Build history of the part. All positions in model axes, mm. A direction names the side the tool comes from. Round coordinates to 2 decimals unless told otherwise and drop trailing zeros. Write each loop counter-clockwise with the first axis right and the second up, starting at its lowest first coordinate (ties: lowest second). Pieces come first, ordered by that corner, then holes.
Item 1: Band-saw the part on D-D, the plane y = -9. Write the cut outline in (x, z).
Item 2: Band-saw the part on C-C, the plane y = -2. Write the cut outline in (x, z), then the cut area to 3 significant figures.
Item 3: Band-saw the part on B-B, the plane z = -55. Write the cut outline in (x, y), then the cut area to 3 significant figures.
Item 4: Band-saw the part on A-A, the plane x = 30. Write the cut outline in (y, z).
Item 5: Mould opens along Z. For faces 1 (the flat face through (17.4, 0.4, 0)), 2 (the cylindrical face through (0.986, -8.512, -86.282)), 3 (the flat face through (22, 1, -17)), 4 (the cylindrical face through (44.1, 1.14, -11.15)) say: +Z half, -Z half, draft (parallel to the pull), parting line (faces both ways), or undercut.
Item 6: Wall check: probe 1 along X at (y, z) = (-11.25, -5); probe 2 along Z at (x, y) = (0.9, -9); probe 3 along Z at (x, y) = (0.95, -9.5). Give the ranges that are in metal, low to high.
Item 7: Drop flat-ended pins along their axis: pin 1 Ø2 at (x, z) = (1, -49.5) entering from +Y; pin 2 Ø0.6 at (x, y) = (22, 1.5) entering from -Z; pin 3 Ø0.6 at (y, z) = (0.5, -14) entering from -X; pin 4 Ø12 at (x, z) = (11, -80) entering from +Y. Give the stop position or say it passes through.
Item 8: 3-axis set-ups, long thin cutter, end or side, ignore diameter. For faces 5 (the cylindrical face through (43.99, -9.12, -56.71)), 6 (the flat face through (2, -7.7, -54.2)), 7 (the cylindrical face through (44.014, -9.867, -93.905)): which of +Z, -Z, +X, -X, +Y, -Y reach the whole face in a straight line?
```python
from build123d import *

# Parameters (mm, degrees)
SKETCH1_W                      = 45
SKETCH1_H                      = 22
BASE_FLANGE1_DEPTH             = 2
EDGE_FLANGE3_STRIP_W           = 10
EDGE_FLANGE3_STRIP_H           = 2
EDGE_FLANGE3_STRIP_CUT_DEPTH   = 22
EDGE_FLANGE3_STRIP_2_W         = 10
EDGE_FLANGE3_STRIP_2_H         = 2
EDGE_FLANGE3_STRIP_CUT_2_DEPTH = 22
EDGE_FLANGE3_DEPTH             = 22
EDGE_FLANGE3_PROFILE_W         = 110
EDGE_FLANGE3_PROFILE_H         = 17
EDGE_FLANGE3_FLAT_DEPTH        = 2
EDGE_FLANGE3_BEND_DEPTH        = 22
EDGE_FLANGE3_PROFILE_2_W       = 110
EDGE_FLANGE3_PROFILE_2_H       = 17
EDGE_FLANGE3_FLAT_2_DEPTH      = 2
SKETCH34_R                     = 4
CUT_EXTRUDE1_DEPTH             = 10
SKETCH35_R                     = 3.75
CUT_EXTRUDE2_DEPTH             = 10
SKETCH36_R                     = 1.75
CUT_EXTRUDE3_DEPTH             = 121.203993278
SKETCH37_W                     = 23
SKETCH37_H                     = 12
CUT_EXTRUDE4_DEPTH             = 10
CHAMFER1_SIZE                  = 2
CHAMFER2_SIZE                  = 10


# Sheet-metal steps are written as plain solids
with BuildPart() as part:
    # Sketch1 → Base-Flange1 (new body)
    with BuildSketch(Plane(origin=(0, 0, 0), x_dir=(1, 0, 0), z_dir=(0, 1, 0))):
        with Locations((22.5, 11)):
            Rectangle(SKETCH1_W, SKETCH1_H)
    extrude(amount=BASE_FLANGE1_DEPTH)

    # Edge-Flange3 strip (across the edge) → Edge-Flange3 strip cut (cut)
    with BuildSketch(Plane(origin=(45, 0, -22), x_dir=(-1, 0, 0), z_dir=(0, 0, 1))):
        with Locations((-2, -1)):
            Rectangle(EDGE_FLANGE3_STRIP_W, EDGE_FLANGE3_STRIP_H)
    extrude(amount=EDGE_FLANGE3_STRIP_CUT_DEPTH, mode=Mode.SUBTRACT)

    # Edge-Flange3 strip 2 (across the edge) → Edge-Flange3 strip cut 2 (cut)
    with BuildSketch(Plane(origin=(0, 0, 0), x_dir=(1, 0, 0), z_dir=(0, 0, -1))):
        with Locations((-2, -1)):
            Rectangle(EDGE_FLANGE3_STRIP_2_W, EDGE_FLANGE3_STRIP_2_H)
    extrude(amount=EDGE_FLANGE3_STRIP_CUT_2_DEPTH, mode=Mode.SUBTRACT)

    # Edge-Flange3 bend section (across the edge) → Edge-Flange3 (add)
    with BuildSketch(Plane(origin=(45, 0, -22), x_dir=(-1, 0, 0), z_dir=(0, 0, 1))):
        with BuildLine():
            Line((0, 1), (2, 1))
            ThreePointArc((2, 1), (2.292893219, 0.292893219), (3, 0))
            Line((3, 0), (3, -2))
            ThreePointArc((3, -2), (0.878679656, -1.121320344), (0, 1))
        make_face()
    extrude(amount=EDGE_FLANGE3_DEPTH)

    # Edge-Flange3 profile (on flange) → Edge-Flange3 flat (add)
    with BuildSketch(Plane(origin=(45, 0, 0), x_dir=(0, 0, 1), z_dir=(1, 0, 0))):
        with Locations((-55, 9.5)):
            Rectangle(EDGE_FLANGE3_PROFILE_W, EDGE_FLANGE3_PROFILE_H)
    extrude(amount=-EDGE_FLANGE3_FLAT_DEPTH)

    # Edge-Flange3 bend section 2 (across the edge) → Edge-Flange3 bend (add)
    with BuildSketch(Plane(origin=(0, 0, 0), x_dir=(1, 0, 0), z_dir=(0, 0, -1))):
        with BuildLine():
            Line((0, 1), (2, 1))
            ThreePointArc((2, 1), (2.292893219, 0.292893219), (3, 0))
            Line((3, 0), (3, -2))
            ThreePointArc((3, -2), (0.878679656, -1.121320344), (0, 1))
        make_face()
    extrude(amount=EDGE_FLANGE3_BEND_DEPTH)

    # Edge-Flange3 profile 2 (on flange) → Edge-Flange3 flat 2 (add)
    with BuildSketch(Plane(origin=(0, 0, 0), x_dir=(0, 0, -1), z_dir=(-1, 0, 0))):
        with Locations((55, 9.5)):
            Rectangle(EDGE_FLANGE3_PROFILE_2_W, EDGE_FLANGE3_PROFILE_2_H)
    extrude(amount=-EDGE_FLANGE3_FLAT_2_DEPTH)

    # Sketch34 → Cut-Extrude1 (cut)
    with BuildSketch(Plane(origin=(45, 0, 0), x_dir=(0, 0, -1), z_dir=(1, 0, 0))):
        with Locations(Location((90, -9, 0), (0, 0, 90))):
            Circle(SKETCH34_R)
    extrude(amount=-CUT_EXTRUDE1_DEPTH, mode=Mode.SUBTRACT)

    # Sketch35 → Cut-Extrude2 (cut)
    with BuildSketch(Plane.ZY):
        with Locations(Location((-90, -9, 0), (0, 0, 270))):
            Circle(SKETCH35_R)
    extrude(amount=-CUT_EXTRUDE2_DEPTH, mode=Mode.SUBTRACT)

    # Sketch36 → Cut-Extrude3 (cut, through all)
    with BuildSketch(Plane.ZY):
        with Locations(Location((-55, -9.5, 0), (0, 0, 270))):
            Circle(SKETCH36_R)
    extrude(amount=-CUT_EXTRUDE3_DEPTH, mode=Mode.SUBTRACT)

    # Sketch37 → Cut-Extrude4 (cut)
    with BuildSketch(Plane(origin=(0, 2, 0), x_dir=(1, 0, 0), z_dir=(0, 1, 0))):
        with Locations((22.5, 11)):
            Rectangle(SKETCH37_W, SKETCH37_H)
    extrude(amount=-CUT_EXTRUDE4_DEPTH, mode=Mode.SUBTRACT)

    # Chamfer1
    chamfer1_edges = [part.edges().sort_by_distance(p)[0] for p in [
        (44, -1, -110),
        (44, -18, -110),
        (1, -1, -110),
        (1, -18, -110),
    ]]
    chamfer(chamfer1_edges, length=CHAMFER1_SIZE)

    # Chamfer2
    chamfer2_edges = [part.edges().sort_by_distance(p)[0] for p in [
        (44, -18, 0),
        (1, -18, 0),
    ]]
    chamfer(chamfer2_edges, length=CHAMFER2_SIZE)


solid = part.part
```
Results:
1. outline: (0, -110) - (2, -110) - (2, -93.75) - (0, -93.75) - close; (0, -86.25) - (2, -86.25) - (2, -56.68) - (0, -56.68) - close; (0, -53.32) - (2, -53.32) - (2, -1) - (0, -1) - close; (43, -110) - (45, -110) - (45, -94) - (43, -94) - close; (43, -86) - (45, -86) - (45, -56.68) - (43, -56.68) - close; (43, -53.32) - (45, -53.32) - (45, -1) - (43, -1) - close
2. outline: (0, -109) - (2, -109) - (2, 0) - (0, 0) - close; (43, -109) - (45, -109) - (45, 0) - (43, 0) - close
2. area: 436 mm2
3. outline: (0, -18) - (2, -18) - (2, -11.25) - (0, -11.25) - close; (0, -7.75) - (2, -7.75) - (2, -1) - (0, -1) - close; (43, -18) - (45, -18) - (45, -11.25) - (43, -11.25) - close; (43, -7.75) - (45, -7.75) - (45, -1) - (43, -1) - close
3. area: 54.0 mm2
4. outline: (0, -22) - (2, -22) - (2, -17) - (0, -17) - close; (0, -5) - (2, -5) - (2, 0) - (0, 0) - close
5. face 1: +Z half
5. face 2: undercut
5. face 3: undercut
5. face 4: draft
6. probe 1: x = 0 to 2, 43 to 45
6. probe 2: z = -110 to -93.75, -86.25 to -56.68, -53.32 to -1
6. probe 3: z = -110 to -93.72, -86.28 to -56.75, -53.25 to -1.5
7. pin 1: stops at y = -1
7. pin 2: stops at z = -22
7. pin 3: stops at x = 0.25
7. pin 4: passes through
8. face 5: +X, -X
8. face 6: +Z, -Z, -Y
8. face 7: +X
